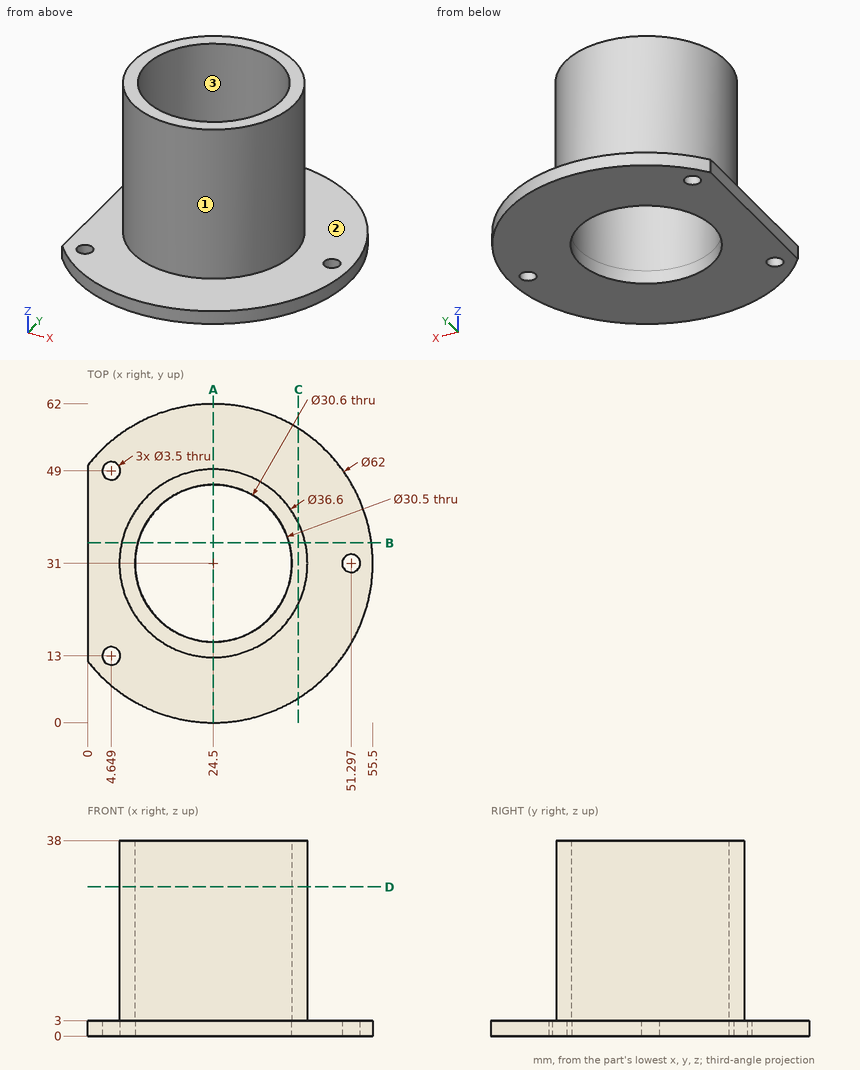
Geometry: see drawing. Coordinates: mm, zero at the bounding-box minimum. Round coordinates to 2 decimals unless told otherwise and drop trailing zeros. Write each loop counter-clockwise with the first axis right and the second up, starting at its lowest first coordinate (ties: lowest second). Pieces come first, ordered by that corner, then holes. Notation, with made-up numbers: M 39.25,13.5 L 62.25,13.5 A27 cw 62.25,41.5 Z; hole C 87.25,52.25 d6. An arc over 180 degrees is marked long. Answer as a JSON object with one key per item and string values. Group by question number.
(1) Section query C-C on x = 41. Output: boundary loops of the cut face in (y, z) (1 decimal).
(2) First-contact query: pin 1 (1.5 mm diameter, centred on y = 19.5, z = 9.5, fed in from -X); pin 2 (12 mm diameter, centred on y = 39.5, z = 12, fed in from +X); pin 3 (1.5 mm diameter, centred on x = 8, y = 42.5, fed in from +Z). Flat tips, straight axial feed; report the tip coordinate or a pass-through.
(3) Ray query, line 1 (Y direction, x = 24.5, z = 16); line 2 (Y direction, x = 24, z = 2); line 3 (Z direction, x = 35, y = 50). Return the intervals inside material, ascending. Write a range as [from, to].
(4) Section query A-A on x = 24.5. Output: boundary loops of the cut face in (y, z).
(5) Mould query, pull axis Y, two halves, no side actions, for the marked faces 1, 2 and 3. Classes: +Y half, -Y half, draft (parallel to the pull), parting line (faces both ways), or undercut.
(6) Section query D-D on z = 29. Output: boundary loops of the cut face in (x, y).
(7) Section query B-B on y = 35. Output: boundary loops of the cut face in (x, z), then the cut area to 3 significant figures.
Computed values:
{
 "1": {"outline": "M 4.8,0 L 57.2,0 L 57.2,3 L 38.9,3 L 38.9,38 L 23.1,38 L 23.1,3 L 4.8,3 Z"},
 "2": {"pin 1": "x = 9.69", "pin 2": "x = 42.63", "pin 3": "z = 3"},
 "3": {"line 1": "[12.7, 15.7], [46.3, 49.3]", "line 2": "[0, 15.76], [46.24, 62]", "line 3": "[0, 3]"},
 "4": {"outline": "M 0,0 L 15.75,0 L 15.75,3 L 15.7,3 L 15.7,38 L 12.7,38 L 12.7,3 L 0,3 Z; M 46.25,0 L 62,0 L 62,3 L 49.3,3 L 49.3,38 L 46.3,38 L 46.3,3 L 46.25,3 Z"},
 "5": {"face 1": "parting line", "face 2": "draft", "face 3": "undercut"},
 "6": {"outline": "C 24.5,31 d36.6; hole C 24.5,31 d30.6"},
 "7": {"outline": "M 0,0 L 9.78,0 L 9.78,3 L 9.73,3 L 9.73,38 L 6.64,38 L 6.64,3 L 0,3 Z; M 39.22,0 L 55.24,0 L 55.24,3 L 42.36,3 L 42.36,38 L 39.27,38 L 39.27,3 L 39.22,3 Z", "area": "294 mm^2"}
}
